Part model, mm, in its own coordinate system. Give positions to 0.01 mm unless a question says otherwise; leave off trailing zeros. Write each loop counter-clockwise with the first axis right and the second up, starting at its lowest first coordinate (ties: lowest second). Pieces come first, ordered by that corner, then holes. Notation, with made-up numbers: M 76,-6 L 96,-6 A6 cw 96,-2 Z; hole C 53,61.25 d9. An arc over 180 degrees is marked long. Use CSV: the item, a comma, the result in double quotes. Start each with the question number.
Item 1: Cut at A-A (y = -51). List the corners of the cut face in (x, z).
Item 2: Drill centre lines: line 1 (X direction, y = 38.5, z = 1.6); line 2 (Y direction, x = -92, z = 1.65). Where is each one in solid material? Low to high. Write a range as [from, to].
Item 3: Pin check, flat tips, straight feed: pin 1 (0.9 mm diameter, centred on x = 2, z = 1, fed in from -Y); pin 2 (0.9 mm diameter, centred on y = 43, z = 1, fed in from +X); pin 3 (1.5 mm diameter, centred on x = -109.5, z = 1, fed in from +Y). Stop position of each tip, or through.
Item 4: Cut at B-B (x = -114.5). List the corners of the cut face in (y, z), then the cut area to 3 significant figures.
from build123d import *

# Parameters (mm, degrees)
SKETCH1_W           = 292
SKETCH1_H           = 151
BOSS_EXTRUDE1_DEPTH = 3
SKETCH2_W           = 35
SKETCH2_H           = 3
CUT_EXTRUDE1_DEPTH  = 3
SKETCH4_W           = 35
SKETCH4_H           = 3
CUT_EXTRUDE2_DEPTH  = 3
SKETCH5_W           = 3
SKETCH5_H           = 35
CUT_EXTRUDE3_DEPTH  = 3
SKETCH7_W           = 3
SKETCH7_H           = 35
CUT_EXTRUDE4_DEPTH  = 3


with BuildPart() as part:
    # Sketch1 → Boss-Extrude1 (new body)
    with BuildSketch(Plane.XY):
        Rectangle(SKETCH1_W, SKETCH1_H)
    extrude(amount=BOSS_EXTRUDE1_DEPTH)

    # Sketch2 → Cut-Extrude1 (cut)
    with BuildSketch(Plane.XY.offset(3)):
        with Locations((103.5, 74)):
            Rectangle(SKETCH2_W, SKETCH2_H)
        with Locations((-103.5, 74)):
            Rectangle(SKETCH2_W, SKETCH2_H)
        with Locations((-103.5, -74)):
            Rectangle(SKETCH2_W, SKETCH2_H)
        with Locations((103.5, -74)):
            Rectangle(SKETCH2_W, SKETCH2_H)
    extrude(amount=-CUT_EXTRUDE1_DEPTH, mode=Mode.SUBTRACT)

    # Sketch4 → Cut-Extrude2 (cut)
    with BuildSketch(Plane.XY):
        with Locations((0, -74)):
            Rectangle(SKETCH4_W, SKETCH4_H)
        with Locations((0, 74)):
            Rectangle(SKETCH4_W, SKETCH4_H)
    extrude(amount=CUT_EXTRUDE2_DEPTH, mode=Mode.SUBTRACT)

    # Sketch5 → Cut-Extrude3 (cut)
    with BuildSketch(Plane(origin=(146, 0, 0), x_dir=(0, 0, -1), z_dir=(1, 0, 0))):
        with Locations((-1.5, -36.45)):
            Rectangle(SKETCH5_W, SKETCH5_H)
        with Locations((-1.5, 36.45)):
            Rectangle(SKETCH5_W, SKETCH5_H)
    extrude(amount=-CUT_EXTRUDE3_DEPTH, mode=Mode.SUBTRACT)

    # Sketch7 → Cut-Extrude4 (cut)
    with BuildSketch(Plane.ZY.offset(146)):
        with Locations((1.5, -36.45)):
            Rectangle(SKETCH7_W, SKETCH7_H)
        with Locations((1.5, 36.45)):
            Rectangle(SKETCH7_W, SKETCH7_H)
    extrude(amount=-CUT_EXTRUDE4_DEPTH, mode=Mode.SUBTRACT)


solid = part.part
Worked answers:
1,outline,"M -143,0 L 143,0 L 143,3 L -143,3 Z"
2,line 1,"x = [-143, 143]"
2,line 2,"y = [-72.5, 72.5]"
3,pin 1,"stops at y = -72.5"
3,pin 2,"stops at x = 143"
3,pin 3,"stops at y = 72.5"
4,outline,"M -72.5,0 L 72.5,0 L 72.5,3 L -72.5,3 Z"
4,area,"435 mm^2"
